```python
from build123d import *

# Parameters (mm, degrees)
SKETCH2_W           = 203.2
SKETCH2_H           = 254
BASE_FLANGE1_DEPTH  = 0.7
EDGE_FLANGE4_DEPTH  = 203.2
EDGE_FLANGE5_DEPTH  = 255
EDGE_FLANGE6_DEPTH  = 255
EDGE_FLANGE7_DEPTH  = 25.4
EDGE_FLANGE9_DEPTH  = 25.4
EDGE_FLANGE10_DEPTH = 101.6
EDGE_FLANGE11_DEPTH = 101.6
SKETCH76_W          = 12.7
SKETCH76_H          = 12.7
TAB1_DEPTH          = 0.7
SKETCH79_W          = 12.7
SKETCH79_H          = 12.7
TAB2_DEPTH          = 0.7
SKETCH86_R          = 3.15
CUT_EXTRUDE3_DEPTH  = 323.546585783


# Sheet-metal steps are written as plain solids
with BuildPart() as part:
    # Sketch2 → Base-Flange1 (new body)
    with BuildSketch(Plane(origin=(0, 0, 0), x_dir=(1, 0, 0), z_dir=(0, 1, 0))):
        Rectangle(SKETCH2_W, SKETCH2_H)
    extrude(amount=-BASE_FLANGE1_DEPTH)

    # Edge-Flange4 section (across the edge) → Edge-Flange4 (add)
    with BuildSketch(Plane(origin=(101.6, 0, -129), x_dir=(0, 0, 1), z_dir=(-1, 0, 0))):
        with BuildLine():
            Line((-0.7, 1), (-0.7, 202.5))
            Line((-0.7, 202.5), (0, 202.5))
            Line((0, 202.5), (0, 1))
            ThreePointArc((0, 1), (0.292893219, 0.292893219), (1, 0))
            Line((1, 0), (2, 0))
            Line((2, 0), (2, -0.7))
            Line((2, -0.7), (1, -0.7))
            ThreePointArc((1, -0.7), (-0.202081528, -0.202081528), (-0.7, 1))
        make_face()
    extrude(amount=EDGE_FLANGE4_DEPTH)

    # Edge-Flange5 section (across the edge) → Edge-Flange5 (add)
    with BuildSketch(Plane(origin=(-103.6, 0, -128), x_dir=(1, 0, 0), z_dir=(0, 0, 1))):
        with BuildLine():
            Line((-0.7, 1), (-0.7, 202.5))
            Line((-0.7, 202.5), (0, 202.5))
            Line((0, 202.5), (0, 1))
            ThreePointArc((0, 1), (0.292893219, 0.292893219), (1, 0))
            Line((1, 0), (2, 0))
            Line((2, 0), (2, -0.7))
            Line((2, -0.7), (1, -0.7))
            ThreePointArc((1, -0.7), (-0.202081528, -0.202081528), (-0.7, 1))
        make_face()
    extrude(amount=EDGE_FLANGE5_DEPTH)

    # Edge-Flange6 section (across the edge) → Edge-Flange6 (add)
    with BuildSketch(Plane(origin=(103.6, 0, 127), x_dir=(-1, 0, 0), z_dir=(0, 0, -1))):
        with BuildLine():
            Line((-0.7, 1), (-0.7, 202.5))
            Line((-0.7, 202.5), (0, 202.5))
            Line((0, 202.5), (0, 1))
            ThreePointArc((0, 1), (0.292893219, 0.292893219), (1, 0))
            Line((1, 0), (2, 0))
            Line((2, 0), (2, -0.7))
            Line((2, -0.7), (1, -0.7))
            ThreePointArc((1, -0.7), (-0.202081528, -0.202081528), (-0.7, 1))
        make_face()
    extrude(amount=EDGE_FLANGE6_DEPTH)

    # Edge-Flange7 section (across the edge) → Edge-Flange7 (add)
    with BuildSketch(Plane(origin=(-103.6, 151.7, -129.8), x_dir=(0, 0, 1), z_dir=(0, 1, 0))):
        with BuildLine():
            Line((-0.7, 1), (-0.7, 24.7))
            Line((-0.7, 24.7), (0, 24.7))
            Line((0, 24.7), (0, 1))
            ThreePointArc((0, 1), (0.292893219, 0.292893219), (1, 0))
            Line((1, 0), (1.8, 0))
            Line((1.8, 0), (1.8, -0.7))
            Line((1.8, -0.7), (1, -0.7))
            ThreePointArc((1, -0.7), (-0.202081528, -0.202081528), (-0.7, 1))
        make_face()
    extrude(amount=EDGE_FLANGE7_DEPTH)

    # Edge-Flange9 section (across the edge) → Edge-Flange9 (add)
    with BuildSketch(Plane(origin=(103.6, 177.1, -129.8), x_dir=(0, 0, 1), z_dir=(0, -1, 0))):
        with BuildLine():
            Line((-0.7, 1), (-0.7, 24.7))
            Line((-0.7, 24.7), (0, 24.7))
            Line((0, 24.7), (0, 1))
            ThreePointArc((0, 1), (0.292893219, 0.292893219), (1, 0))
            Line((1, 0), (1.8, 0))
            Line((1.8, 0), (1.8, -0.7))
            Line((1.8, -0.7), (1, -0.7))
            ThreePointArc((1, -0.7), (-0.202081528, -0.202081528), (-0.7, 1))
        make_face()
    extrude(amount=EDGE_FLANGE9_DEPTH)

    # Edge-Flange10 section (across the edge) → Edge-Flange10 (add)
    with BuildSketch(Plane(origin=(103.6, 75.5, 128.8), x_dir=(0, 0, -1), z_dir=(0, 1, 0))):
        with BuildLine():
            Line((-0.7, 1), (-0.7, 10))
            Line((-0.7, 10), (0, 10))
            Line((0, 10), (0, 1))
            ThreePointArc((0, 1), (0.292893219, 0.292893219), (1, 0))
            Line((1, 0), (1.8, 0))
            Line((1.8, 0), (1.8, -0.7))
            Line((1.8, -0.7), (1, -0.7))
            ThreePointArc((1, -0.7), (-0.202081528, -0.202081528), (-0.7, 1))
        make_face()
    extrude(amount=EDGE_FLANGE10_DEPTH)

    # Edge-Flange11 section (across the edge) → Edge-Flange11 (add)
    with BuildSketch(Plane(origin=(-103.6, 177.1, 128.8), x_dir=(0, 0, -1), z_dir=(0, -1, 0))):
        with BuildLine():
            Line((-0.7, 1), (-0.7, 10))
            Line((-0.7, 10), (0, 10))
            Line((0, 10), (0, 1))
            ThreePointArc((0, 1), (0.292893219, 0.292893219), (1, 0))
            Line((1, 0), (1.8, 0))
            Line((1.8, 0), (1.8, -0.7))
            Line((1.8, -0.7), (1, -0.7))
            ThreePointArc((1, -0.7), (-0.202081528, -0.202081528), (-0.7, 1))
        make_face()
    extrude(amount=EDGE_FLANGE11_DEPTH)

    # Sketch76 → Tab1 (add)
    with BuildSketch(Plane.ZY.offset(104.3)):
        with Locations((133.35, 8.35)):
            Rectangle(SKETCH76_W, SKETCH76_H)
    extrude(amount=-TAB1_DEPTH)

    # Sketch79 → Tab2 (add)
    with BuildSketch(Plane(origin=(104.3, 0, 0), x_dir=(0, 0, -1), z_dir=(1, 0, 0))):
        with Locations((-133.35, 8.35)):
            Rectangle(SKETCH79_W, SKETCH79_H)
    extrude(amount=-TAB2_DEPTH)

    # Sketch86 → Cut-Extrude3 (cut, through all)
    with BuildSketch(Plane(origin=(104.3, 0, 0), x_dir=(0, 0, -1), z_dir=(1, 0, 0))):
        with Locations(Location((-133.35, 8.35, 0), (0, 0, 90))):
            Circle(SKETCH86_R)
    extrude(amount=-CUT_EXTRUDE3_DEPTH, mode=Mode.SUBTRACT)


solid = part.part
```
Work out the finished part from the listing and answer in its coordinate system (mm). A direction names the side the tool comes from. Give positions to 0.01 mm unless a question says otherwise; leave off trailing zeros. Order: outer loops, then holes, each group sorted by start corner. A loop starts at its lowest first (then second) coordinate and runs counter-clockwise, first axis right, second up.
1. The mould has two halves that part along Y. Classify faces 3 (the flat face through (-1, -0.7, 1)), 4 (the cylindrical face through (-103.945, 7.94, 136.473)), 5 (the flat face through (98, 126, 129.5)), 6 (the flat face through (1, 0, 1)): released by +Y, released by -Y, zero draft, split by the parting line, or undercut.
Result sheet:
face 3: released by -Y
face 4: undercut
face 5: zero draft
face 6: released by +Y
2. Section B-B, the plane x = -6.5 is taken. Determine the outline of the cut face in (y, z).
Result sheet:
outline: (-0.7, -128) arc R1.7 ccw to (1, -129.7) - (202.5, -129.7) - (202.5, -129) - (1, -129) arc R1 cw to (0, -128) - (0, 127) - (-0.7, 127) - close
3. Section C-C, the plane z = -110 is taken. Determine the outline of the cut face in (x, y).
Result sheet:
outline: (-104.3, 1) arc R1.7 ccw to (-102.6, -0.7) - (102.6, -0.7) arc R1.7 ccw to (104.3, 1) - (104.3, 202.5) - (103.6, 202.5) - (103.6, 1) arc R1 cw to (102.6, 0) - (-102.6, 0) arc R1 cw to (-103.6, 1) - (-103.6, 202.5) - (-104.3, 202.5) - close
4. Straight lines are drawn through the part: L1, parallel to Y at x = 103.95, z = 133.35; L2, parallel to X at y = 42, z = 63; L3, parallel to Z at x = -104, y = 8.35. For each, find the intervals that lie inside material, in ascending order.
Result sheet:
L1: y = 2 to 5.2, 11.5 to 14.7
L2: x = -104.3 to -103.6, 103.6 to 104.3
L3: z = -128 to 130.2, 136.5 to 139.7
5. Section A-A, the plane y = 46 is taken. Determine the outline of the cut face in (x, z), and give its area (3 significant figures).
Result sheet:
outline: (-104.3, -128) - (-103.6, -128) - (-103.6, 127) - (-104.3, 127) - close; (-101.6, -129.7) - (101.6, -129.7) - (101.6, -129) - (-101.6, -129) - close; (103.6, -128) - (104.3, -128) - (104.3, 127) - (103.6, 127) - close
area: 499 mm2
6. For faces 1 (the flat face through (98, 126, 128.8)), 2 (the flat face through (-104.3, 100, 4)), determine the directions among +Z, -Z, +X, -X, +Y, -Y from which every point of the face is accessible in a straight line to the end or side of a thin tool.
Result sheet:
face 1: +Y, -Y
face 2: +Z, -Z, -X, +Y, -Y
7. Each of these flat-tipped pins is pushed along its axis until it touches: P1, Ø0.5, axis at y = 144, z = -129, coming from the -X side; P2, Ø6, axis at x = -49.5, z = 2, coming from the +Y side; P3, Ø0.6, axis at x = -104, y = 183.5, coming from the +Z side. Where does it stop, or does it pass through?
Result sheet:
P1: stops at x = -101.6
P2: stops at y = 0
P3: stops at z = 127
